Here's how the part is built. I have some questions about the finished solid (model axes, mm). A direction names the side the tool comes from. Coordinates: 2 decimals unless noted, no trailing zeros. Write each loop counter-clockwise with the first axis right and the second up, starting at its lowest first coordinate (ties: lowest second). Pieces come first, ordered by that corner, then holes.
Item 1: If I drill on line 1 (Y direction, x = 39.5, z = 29); line 2 (X direction, y = 40, z = 52), over which ranges is the centre line in solid material (lowest first)?
Item 2: If we section it at A-A (z = 24): Please give me the cut outline in (x, y), then the cut area to 3 significant figures.
Item 3: We'd pull the mould along X, two halves only. Please class faces 5 (the face through (45, 25, 15)), 6 (the face through (25, 0, 24)), 7 (the face through (42, 25, 62)): +X half, -X half, draft (parallel to the pull), parting line (faces both ways), or undercut.
Item 4: For faces 1 (the face through (8, 25, 62)), 2 (the face through (25, 8, 62)), 3 (the face through (25, 42, 62)), 4 (the face through (25, 45, 15)), which set-ups out of +Z, -Z, +X, -X, +Y, -Y let a thin tool reach every point of the face, with its end or its side?
Item 5: I'm going to push flat-ended pins straight in: pin 1 Ø22.5 at (y, z) = (18.5, 59.5) entering from -X; pin 2 Ø2 at (x, z) = (17.5, 53) entering from -Y; pin 3 Ø12 at (x, y) = (17, 24) entering from -Z; pin 4 Ø1 at (x, z) = (43, 53.5) entering from -Y. Where does each tip first touch, or does it pass through?
Item 6: If we section it at D-D (z = 69): Please give me the cut outline in (x, y).
Item 7: If we section it at B-B (x = 30): Please give me the cut outline in (y, z).
from build123d import *

# Parameters (mm, degrees)
F0_W     = 50
F0_H     = 50
F0_W_2   = 40
F0_H_2   = 40
F1_DEPTH = 30
F2_W     = 50
F2_H     = 50
F3_DEPTH = 18
F4_W     = 34
F4_H     = 34
F5_DEPTH = 33
F6_R     = 5


with BuildPart() as f1:
    # F0 (on Top) → F1 (new body)
    with BuildSketch(Plane.XY):
        with Locations((25, 25)):
            Rectangle(F0_W, F0_H)
        with Locations((25, 25)):
            Rectangle(F0_W_2, F0_H_2, mode=Mode.SUBTRACT)
    extrude(amount=F1_DEPTH)

    # F2 (on face) → F3 (join)
    with BuildSketch(Plane.XY.offset(30)):
        with Locations((25, 25)):
            Rectangle(F2_W, F2_H)
    extrude(amount=F3_DEPTH)

    # F4 (on face) → F5 (join)
    with BuildSketch(Plane.XY.offset(48)):
        with Locations((25, 25)):
            Rectangle(F4_W, F4_H)
    extrude(amount=F5_DEPTH)

    # F6
    f6_edges = [f1.edges().sort_by_distance(p)[0] for p in [
        (25, 8, 81),
        (8, 25, 81),
        (25, 42, 81),
        (42, 25, 81),
    ]]
    fillet(f6_edges, radius=F6_R)


solid = f1.part
Answer list:
1. line 1: y = 0 to 5, 45 to 50
1. line 2: x = 8 to 42
2. outline: (0, 0) - (50, 0) - (50, 50) - (0, 50) - close; hole (5, 5) - (45, 5) - (45, 45) - (5, 45) - close
2. area: 900 mm2
3. face 5: undercut
3. face 6: draft
3. face 7: +X half
4. face 1: +Z, -X, +Y, -Y
4. face 2: +Z, +X, -X, -Y
4. face 3: +Z, +X, -X, +Y
4. face 4: -Z
5. pin 1: stops at x = 8
5. pin 2: stops at y = 8
5. pin 3: stops at z = 30
5. pin 4: passes through
6. outline: (8, 8) - (42, 8) - (42, 42) - (8, 42) - close
7. outline: (0, 0) - (5, 0) - (5, 30) - (45, 30) - (45, 0) - (50, 0) - (50, 48) - (42, 48) - (42, 76) arc R5 ccw to (37, 81) - (13, 81) arc R5 ccw to (8, 76) - (8, 48) - (0, 48) - close
